Verification items for this drawing (mm, ordinates from the low corner). A direction names the side the tool comes from. Coordinates: 2 decimals unless noted, no trailing zeros. Order: outer loops, then holes, each group sorted by start corner. A loop starts at its lowest first (then second) coordinate and runs counter-clockwise, first axis right, second up. Notation, with made-up numbers: M 83,73 L 97,73 A30 ccw 97,98 Z; hole C -8.5,-29.75 d7. An arc over 180 degrees is marked long. Answer as a JSON object with one key per item and string values. Group by question number.
(1) Mould release check, pull along X, two halves, no side actions. Record for the marked faces 6 and 7: released by +X, released by -X, zero draft, split by the parting line, or undercut.
(2) Material ranges on line 1 (X direction, y = 4.5, z = 28.5); line 2 (Z direction, x = 31, y = 4.55); line 3 (Z direction, x = 29, y = 1.5), recorded low to high.
(3) Cross-section at C-C (z = 28). Enter the section's corners in (x, y).
(4) Access from +Z, -Z, +X, -X, +Y, -Y to the whole of each face (thin tool, end or side, straight path). Record for the marked faces 1, 2, 3, 4 and 5.
(5) Gauge pin test, flat ends, axial feed: pin 1 Ø5 at (x, z) = (5, 5) entering from +Y; pin 2 Ø2 at (y, z) = (1, 9) entering from +X; pin 3 Ø0.7 at (y, z) = (5, 22) entering from -X; pin 4 Ø0.6 at (x, y) = (7, 0.5) entering from +Z. Record the tip position at first contact, or that the pin passes through.
(6) Cross-section at A-A (y = 5.25). Enter the section's corners in (x, z).
(7) Cross-section at B-B (x = 18). Enter the section's corners in (y, z).
(8) Cross-section at D-D (x = 32.5). Enter the section's corners in (y, z).
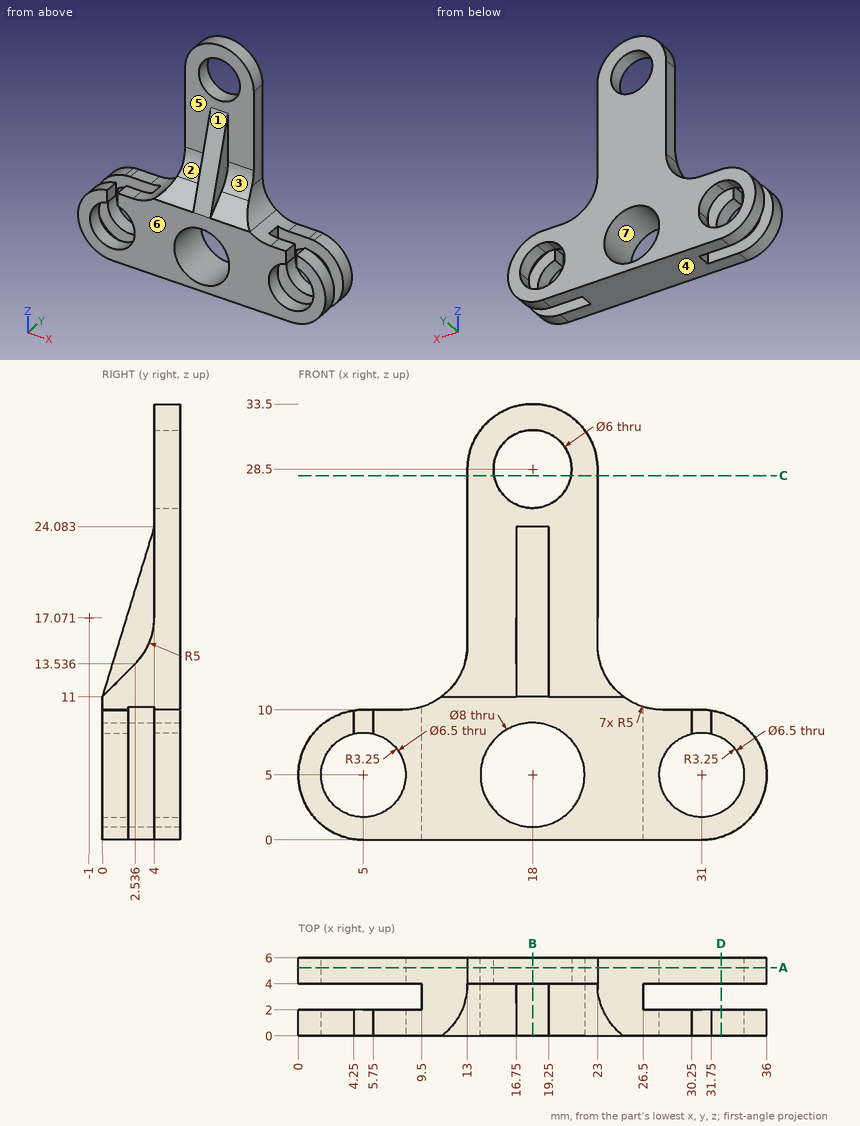
Taken from the geometry:
{
 "1": {"face 6": "zero draft", "face 7": "undercut"},
 "2": {"line 1": "x = 13 to 15, 21 to 23", "line 2": "z = 0 to 1.75, 8.25 to 10", "line 3": "z = 0 to 2.44, 7.56 to 10"},
 "3": {"outline": "M 13,4 L 15.04,4 L 15.04,6 L 13,6 Z; M 20.96,4 L 23,4 L 23,6 L 20.96,6 Z"},
 "4": {"face 1": "+Z, +X, -X, -Y", "face 2": "+Z, -X, -Y", "face 3": "+Z, +X, -Y", "face 4": "-Z, +X, -X, +Y, -Y", "face 5": "+Z, -Y"},
 "5": {"pin 1": "passes through", "pin 2": "stops at x = 35", "pin 3": "stops at x = 13", "pin 4": "stops at z = 10"},
 "6": {"outline": "M 4.25,9.94 A5 ccw 5,0 L 31,0 A5 ccw 31.75,9.94 A5 ccw 31,10 L 28,10 A5 cw 25,11 A5 cw 23,15 L 23,28.5 A5 ccw 13,28.5 L 13,15 A5 cw 11,11 A5 cw 8,10 L 5,10 A5 ccw Z; hole M 4.25,8.16 A3.25 ccw long 5.75,8.16 A3.25 ccw Z; hole C 18,5 d8; hole C 18,28.5 d6; hole M 30.25,8.16 A3.25 ccw long 31.75,8.16 A3.25 ccw Z"},
 "7": {"outline": "M 0,0 L 6,0 L 6,1 L 0,1 Z; M 0,9 L 6,9 L 6,25.5 L 4,25.5 L 4,24.08 L 0,11 Z; M 4,31.5 L 6,31.5 L 6,33.5 L 4,33.5 Z"},
 "8": {"outline": "M 0,0.23 L 2,0.23 L 2,2.12 L 0,2.12 Z; M 0,7.88 L 2,7.88 L 2,9.77 L 0,9.77 Z; M 4,0.23 L 6,0.23 L 6,2.12 L 4,2.12 Z; M 4,7.88 L 6,7.88 L 6,9.77 L 4,9.77 Z"}
}
